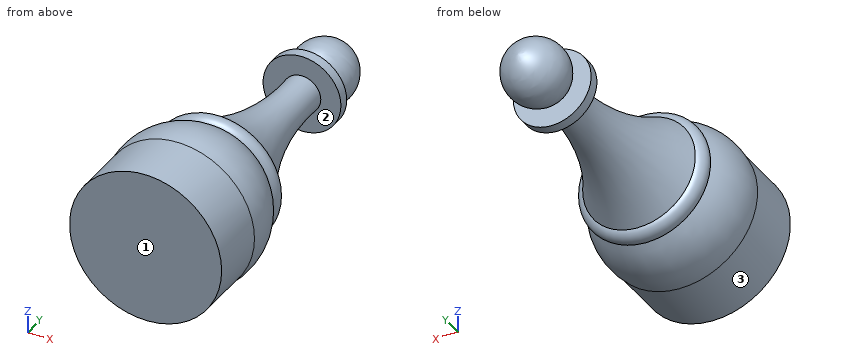
Autodesk Inventor part; units mm, degrees
ref_plane "YZ Plane" through (0, 0, 0) normal (1, 0, 0) x (0, 1, 0)
ref_plane "XZ Plane" through (0, 0, 0) normal (0, 1, 0) x (-1, 0, 0)
ref_plane "XY Plane" through (0, 0, 0) normal (0, 0, 1) x (1, 0, 0)
sketch "Boceto1" plane through (0, 0, 0) normal (0, 0, 1) x (1, 0, 0)
  line L0 (0, 0) -> (0, 50)
  line L1 (12.9556, 0) -> (0, 0)
  arc A0 (2.2833, 41.1879) -> (0, 50) centre (-0.2888, 45.2233) ccw
  line L2 (2.2833, 41.1879) -> (5.5239, 41.1879)
  line L3 (5.5239, 41.1879) -> (5.5239, 39.7245)
  line L4 (5.5239, 39.7245) -> (2.6625, 39.7245)
  arc A1 (2.6625, 39.7245) -> (7.9966, 19.1386) centre (38.2928, 37.9727) ccw
  arc A2 (8.6471, 16.6281) -> (7.9966, 19.1386) centre (7.7402, 17.7327) ccw
  arc A3 (10.796, 8.3345) -> (8.6471, 16.6281) centre (1.334, 10.308) ccw
  line L5 (10.796, 8.3345) -> (10.796, 0)
  dimension "d0" = 50
revolve "Revolución1" add sketch "Boceto1" angle 360 about axis through (0, 0, 0) along (0, 1, 0)
properties part number "PAWN"
The model under review builds one solid part; all positions refer to its coordinate system, in mm. Face numbers are marked on the shaded views. Round coordinates to 2 decimals unless told otherwise and drop trailing zeros. Loops run counter-clockwise (first coordinate to the right, second up) from the corner with the lowest first, then second, coordinate; pieces in that order, holes last. Notation, with made-up numbers: M -34,84.5 L -26,84.5 A8 cw -26,93.5 Z; hole C 41.5,38 d2. An arc over 180 degrees is marked long. Write item = value, one per line.
Item 1: Insertion check: P1, Ø6, axis at x = 6, z = -1, coming from the +Y side; P2, Ø10, axis at y = 21, z = 0, coming from the -X side; P3, Ø4, axis at y = 38, z = 0, coming from the +X side. Each pin has a flat end and moves straight along its axis. Give the tip position at first contact, or say it passes through.
Return value:
P1 = 48.62
P2 = -9.17
P3 = 5.52
Item 2: The part is to be moulded in two halves that separate along Y. For the marked faces 1, 2 and 3, say which applies: released by +Y, released by -Y, zero draft, split by the parting line, or undercut.
Return value:
face_1 = released by -Y
face_2 = undercut
face_3 = zero draft
Item 3: Take a section at C-C on y = 21. Write out the cut boundary in (x, z), then the cut area to 3 significant figures.
Return value:
outline = C 0,0 d13.83
area = 150 mm2
Item 4: Take a section at B-B on z = 4. State how many separate pieces and enclosed holes the cut face has, then the cut area to 3 significant figures.
Return value:
separate_pieces = 3
enclosed_holes = 0
area = 462 mm2
Item 5: For line 1 (Z direction, x = -4.5, y = 23.5); line 2 (Y direction, x = 8, z = -0.5) (3 decimals); line 3 (Z direction, x = 1.5, y = 3), list the stretches that pass through material, from the lowest coordinate up. Write a range as [from, to].
Return value:
line_1 = [-3.48, 3.48]
line_2 = [0, 19.135]
line_3 = [-10.69, 10.69]
Item 6: Take a section at A-A on y = 40.5. Write out the cut boundary in (x, z), then the cut area to 3 significant figures.
Return value:
outline = C 0,0 d11.05
area = 95.9 mm2
